```python
from build123d import *

# Parameters (mm, degrees)
SKETCH2_R           = 1.35
BOSS_EXTRUDE1_DEPTH = 36
CIRPATTERN1_COUNT   = 6
CUT_EXTRUDE3_DEPTH  = 36
CUT_EXTRUDE9_DEPTH  = 36


with BuildPart() as part:
    # Sketch2 → Boss-Extrude1 (new body)
    # profile 1 of 10: a face of its own
    with BuildSketch(Plane(origin=(0, 0, 0), x_dir=(1, 0, 0), z_dir=(0, 1, 0))):
        Polygon((-79.212456933, 112.8), (-56.712456933, 73.82885683), (-35.58143708, 86.02885683), (-58.08143708, 125), (0, 125), (0, 0), (-108.253175473, 62.5), align=None)
        with Locations((-77.887328063, 104.904809472)):
            Circle(SKETCH2_R, mode=Mode.SUBTRACT)
        with Locations((-69.387328063, 90.182377607)):
            Circle(SKETCH2_R, mode=Mode.SUBTRACT)
        with Locations((-43.40656595, 105.182377607)):
            Circle(SKETCH2_R, mode=Mode.SUBTRACT)
        with Locations((-51.90656595, 119.904809472)):
            Circle(SKETCH2_R, mode=Mode.SUBTRACT)
        with Locations((-34.90656595, 90.459945743)):
            Circle(SKETCH2_R, mode=Mode.SUBTRACT)
        with Locations((-60.887328063, 75.459945743)):
            Circle(SKETCH2_R, mode=Mode.SUBTRACT)
        with Locations((-52.108162939, 73.253985699)):
            Circle(SKETCH2_R, mode=Mode.SUBTRACT)
        with Locations((-37.385731074, 81.753985699)):
            Circle(SKETCH2_R, mode=Mode.SUBTRACT)
    # profile 2 of 10: a face of its own
    with BuildSketch(Plane(origin=(0, 0, 0), x_dir=(1, 0, 0), z_dir=(0, 1, 0))):
        with Locations((-77.887328063, 104.904809472)):
            Circle(SKETCH2_R)
    # profile 3 of 10: a face of its own
    with BuildSketch(Plane(origin=(0, 0, 0), x_dir=(1, 0, 0), z_dir=(0, 1, 0))):
        with Locations((-69.387328063, 90.182377607)):
            Circle(SKETCH2_R)
    # profile 4 of 10: a face of its own
    with BuildSketch(Plane(origin=(0, 0, 0), x_dir=(1, 0, 0), z_dir=(0, 1, 0))):
        with Locations((-43.40656595, 105.182377607)):
            Circle(SKETCH2_R)
    # profile 5 of 10: a face of its own
    with BuildSketch(Plane(origin=(0, 0, 0), x_dir=(1, 0, 0), z_dir=(0, 1, 0))):
        with Locations((-34.90656595, 90.459945743)):
            Circle(SKETCH2_R)
    # profile 6 of 10: a face of its own
    with BuildSketch(Plane(origin=(0, 0, 0), x_dir=(1, 0, 0), z_dir=(0, 1, 0))):
        with Locations((-37.385731074, 81.753985699)):
            Circle(SKETCH2_R)
    # profile 7 of 10: a face of its own
    with BuildSketch(Plane(origin=(0, 0, 0), x_dir=(1, 0, 0), z_dir=(0, 1, 0))):
        with Locations((-52.108162939, 73.253985699)):
            Circle(SKETCH2_R)
    # profile 8 of 10: a face of its own
    with BuildSketch(Plane(origin=(0, 0, 0), x_dir=(1, 0, 0), z_dir=(0, 1, 0))):
        with Locations((-60.887328063, 75.459945743)):
            Circle(SKETCH2_R)
    # profile 9 of 10: a face of its own
    with BuildSketch(Plane(origin=(0, 0, 0), x_dir=(1, 0, 0), z_dir=(0, 1, 0))):
        with Locations((-51.90656595, 119.904809472)):
            Circle(SKETCH2_R)
    # profile 10 of 10: a face of its own
    with BuildSketch(Plane(origin=(0, 0, 0), x_dir=(1, 0, 0), z_dir=(0, 1, 0))):
        Polygon((-79.212456933, 112.8), (-58.08143708, 125), (-35.58143708, 86.02885683), (-56.712456933, 73.82885683), align=None)
    boss_extrude1 = extrude(amount=BOSS_EXTRUDE1_DEPTH)

    # CirPattern1: Boss-Extrude1 ×6 about axis
    cirpattern1_axis = Axis((0, 0, 0), (0, 1, 0))
    for i in range(1, CIRPATTERN1_COUNT):
        add(boss_extrude1.rotate(cirpattern1_axis, i * 360 / CIRPATTERN1_COUNT))

    # Sketch4 → Cut-Extrude3 (cut)
    with BuildSketch(Plane(origin=(0, 36, 0), x_dir=(1, 0, 0), z_dir=(0, 1, 0))):
        with BuildLine():
            Line((79.212456933, -112.8), (137.293894013, -12.2))
            ThreePointArc((137.293894013, -12.2), (125.5592118, -23.716902798), (109.56410095, -27.524558982))
            ThreePointArc((109.56410095, -27.524558982), (77.942286341, -45), (78.619017782, -81.123015275))
            ThreePointArc((78.619017782, -81.123015275), (83.319046223, -96.879015699), (79.212456933, -112.8))
        make_face()
        with BuildLine():
            Line((137.293894013, 12.2), (79.212456933, 112.8))
            ThreePointArc((79.212456933, 112.8), (83.319046223, 96.879015699), (78.619017782, 81.123015275))
            ThreePointArc((78.619017782, 81.123015275), (77.942286341, 45), (109.56410095, 27.524558982))
            ThreePointArc((109.56410095, 27.524558982), (125.5592118, 23.716902798), (137.293894013, 12.2))
        make_face()
        with BuildLine():
            Line((58.08143708, 125), (-58.08143708, 125))
            ThreePointArc((-58.08143708, 125), (-42.240165578, 120.595918497), (-30.945083169, 108.647574257))
            ThreePointArc((-30.945083169, 108.647574257), (0, 90), (30.945083169, 108.647574257))
            ThreePointArc((30.945083169, 108.647574257), (42.240165578, 120.595918497), (58.08143708, 125))
        make_face()
        with BuildLine():
            Line((-79.212456933, 112.8), (-137.293894013, 12.2))
            ThreePointArc((-137.293894013, 12.2), (-125.5592118, 23.716902798), (-109.56410095, 27.524558982))
            ThreePointArc((-109.56410095, 27.524558982), (-77.942286341, 45), (-78.619017782, 81.123015275))
            ThreePointArc((-78.619017782, 81.123015275), (-83.319046223, 96.879015699), (-79.212456933, 112.8))
        make_face()
        with BuildLine():
            Line((-137.293894013, -12.2), (-79.212456933, -112.8))
            ThreePointArc((-79.212456933, -112.8), (-83.319046223, -96.879015699), (-78.619017782, -81.123015275))
            ThreePointArc((-78.619017782, -81.123015275), (-77.942286341, -45), (-109.56410095, -27.524558982))
            ThreePointArc((-109.56410095, -27.524558982), (-125.5592118, -23.716902798), (-137.293894013, -12.2))
        make_face()
        with BuildLine():
            Line((-58.08143708, -125), (58.08143708, -125))
            ThreePointArc((58.08143708, -125), (42.240165578, -120.595918497), (30.945083169, -108.647574257))
            ThreePointArc((30.945083169, -108.647574257), (0, -90), (-30.945083169, -108.647574257))
            ThreePointArc((-30.945083169, -108.647574257), (-42.240165578, -120.595918497), (-58.08143708, -125))
        make_face()
    extrude(amount=-CUT_EXTRUDE3_DEPTH, mode=Mode.SUBTRACT)

    # Sketch9 → Cut-Extrude9 (cut)
    with BuildSketch(Plane(origin=(0, 36, 0), x_dir=(1, 0, 0), z_dir=(0, 1, 0))):
        with BuildLine():
            ThreePointArc((-30.945083169, 108.647574257), (-41.549939601, 120.167433406), (-56.457326868, 124.956999109))
            ThreePointArc((-56.457326868, 124.956999109), (-49.371438692, 122.503896044), (-44.358314608, 116.927507176))
            ThreePointArc((-44.358314608, 116.927507176), (-25.945860566, 97.258774942), (-5e-08, 90))
            ThreePointArc((-5e-08, 90), (-18.064676866, 95.022217398), (-30.945083169, 108.647574257))
        make_face()
        with BuildLine():
            ThreePointArc((-79.083034312, 96.879180908), (-81.405766691, 104.008868151), (-79.987272175, 111.371978852))
            ThreePointArc((-79.987272175, 111.371978852), (-83.293080236, 96.067019923), (-78.619017782, 81.123015275))
            ThreePointArc((-78.619017782, 81.123015275), (-73.259315749, 63.155577296), (-77.942286796, 44.999999212))
            ThreePointArc((-77.942286796, 44.999999212), (-71.255639547, 71.099161364), (-79.083034312, 96.879180908))
        make_face()
        with BuildLine():
            ThreePointArc((44.358314608, 116.927507176), (49.371438692, 122.503896044), (56.457326868, 124.956999109))
            ThreePointArc((56.457326868, 124.956999109), (41.549939601, 120.167433406), (30.945083169, 108.647574257))
            ThreePointArc((30.945083169, 108.647574257), (18.064676823, 95.022217372), (-5e-08, 90))
            ThreePointArc((-5e-08, 90), (25.945860523, 97.258774916), (44.358314608, 116.927507176))
        make_face()
        with BuildLine():
            ThreePointArc((-109.56410095, 27.524558982), (-124.843019837, 24.100413483), (-136.444599043, 13.585020257))
            ThreePointArc((-136.444599043, 13.585020257), (-130.777205383, 18.495027893), (-123.44134892, 20.048326268))
            ThreePointArc((-123.44134892, 20.048326268), (-97.201500501, 26.159612891), (-77.942286796, 44.999999212))
            ThreePointArc((-77.942286796, 44.999999212), (-91.323993, 31.866639414), (-109.56410095, 27.524558982))
        make_face()
        with BuildLine():
            ThreePointArc((78.619017782, 81.123015275), (83.293080236, 96.067019923), (79.987272175, 111.371978852))
            ThreePointArc((79.987272175, 111.371978852), (81.405766691, 104.008868151), (79.083034312, 96.879180908))
            ThreePointArc((79.083034312, 96.879180908), (71.255639156, 71.099143577), (77.942304587, 44.999968396))
            ThreePointArc((77.942304587, 44.999968396), (73.259315415, 63.155559508), (78.619017782, 81.123015275))
        make_face()
        with BuildLine():
            ThreePointArc((-123.44134892, -20.048326268), (-130.777205383, -18.495027893), (-136.444599043, -13.585020258))
            ThreePointArc((-136.444599043, -13.585020258), (-124.843019837, -24.100413483), (-109.56410095, -27.524558982))
            ThreePointArc((-109.56410095, -27.524558982), (-91.323992191, -31.866639861), (-77.942285871, -45.000000813))
            ThreePointArc((-77.942285871, -45.000000813), (-97.20149969, -26.159613335), (-123.44134892, -20.048326268))
        make_face()
        with BuildLine():
            ThreePointArc((123.44134892, 20.048326268), (130.777205383, 18.495027893), (136.444599043, 13.585020258))
            ThreePointArc((136.444599043, 13.585020258), (124.843019837, 24.100413483), (109.56410095, 27.524558982))
            ThreePointArc((109.56410095, 27.524558982), (91.324008572, 31.866630809), (77.942304587, 44.999968396))
            ThreePointArc((77.942304587, 44.999968396), (97.2015161, 26.159604336), (123.44134892, 20.048326268))
        make_face()
        with BuildLine():
            ThreePointArc((-78.619017782, -81.123015275), (-83.293080236, -96.067019923), (-79.987272175, -111.371978852))
            ThreePointArc((-79.987272175, -111.371978852), (-81.405766691, -104.008868151), (-79.083034312, -96.879180908))
            ThreePointArc((-79.083034312, -96.879180908), (-71.255639567, -71.099162289), (-77.942285871, -45.000000813))
            ThreePointArc((-77.942285871, -45.000000813), (-73.259315766, -63.15557822), (-78.619017782, -81.123015275))
        make_face()
        with BuildLine():
            ThreePointArc((109.56410095, -27.524558982), (124.843019837, -24.100413483), (136.444599043, -13.585020257))
            ThreePointArc((136.444599043, -13.585020257), (130.777205383, -18.495027893), (123.44134892, -20.048326268))
            ThreePointArc((123.44134892, -20.048326268), (97.201499744, -26.159613306), (77.942285932, -45.000000707))
            ThreePointArc((77.942285932, -45.000000707), (91.323992244, -31.866639831), (109.56410095, -27.524558982))
        make_face()
        with BuildLine():
            ThreePointArc((-44.358314608, -116.927507176), (-49.371438692, -122.503896044), (-56.457326868, -124.956999109))
            ThreePointArc((-56.457326868, -124.956999109), (-41.549939601, -120.167433406), (-30.945083169, -108.647574257))
            ThreePointArc((-30.945083169, -108.647574257), (-18.064676844, -95.022217385), (0, -90))
            ThreePointArc((0, -90), (-25.945860545, -97.258774929), (-44.358314608, -116.927507176))
        make_face()
        with BuildLine():
            ThreePointArc((79.083034312, -96.879180908), (81.405766691, -104.008868151), (79.987272175, -111.371978852))
            ThreePointArc((79.987272175, -111.371978852), (83.293080236, -96.067019923), (78.619017782, -81.123015275))
            ThreePointArc((78.619017782, -81.123015275), (73.259315765, -63.155578159), (77.942285932, -45.000000707))
            ThreePointArc((77.942285932, -45.000000707), (71.255639566, -71.099162227), (79.083034312, -96.879180908))
        make_face()
        with BuildLine():
            ThreePointArc((30.945083169, -108.647574257), (41.549939601, -120.167433406), (56.457326867, -124.956999109))
            ThreePointArc((56.457326867, -124.956999109), (49.371438692, -122.503896044), (44.358314608, -116.927507176))
            ThreePointArc((44.358314608, -116.927507176), (25.945860545, -97.258774929), (0, -90))
            ThreePointArc((0, -90), (18.064676844, -95.022217385), (30.945083169, -108.647574257))
        make_face()
    extrude(amount=-CUT_EXTRUDE9_DEPTH, mode=Mode.SUBTRACT)


solid = part.part
```
Geometry: final body of the model. Coordinates: model frame, mm. A direction names the side the tool comes from. Coordinates: 2 decimals unless noted, no trailing zeros. Loops run counter-clockwise (first coordinate to the right, second up) from the corner with the lowest first, then second, coordinate; pieces in that order, holes last. Notation, with made-up numbers: (79.25, 31) -> (125.25, 31) arc R29 cw to (125.25, 62) -> close; hole circle Ø8 at (-32, 28). An arc over 180 degrees is marked (long way). Use a Markdown table: item, result. Add a question column.
(1) Line query: line 1 along Z through (x, y) = (-78, 10.5); line 2 along X through (y, z) = (21, -67.5); line 3 along Z through (x, y) = (-121, 7.5). Output: solid intervals per line, ascending.
(2) Access query for faces 5 (the cylindrical face through (-81.41, 18.25, 104.11)), 6 (the cylindrical face through (-49.283, 18.252, 122.445)), 7 (the cylindrical face through (-49.46, 18.25, -122.56)). Directions: +Z, -Z, +X, -X, +Y, -Y. A direction counts if a zero-diameter tool reaches every point of the face in a straight line with its end or side. Return the directions, or none.
(3) Pin query (flat end, axial travel): pin 1 Ø10 at (y, z) = (10, 59.5) entering from +X; pin 2 Ø10 at (x, y) = (-27, 9) entering from +Z; pin 3 Ø2 at (x, y) = (-13.5, 23.5) entering from -Z. Return the tip coordinate at first contact, or that it passes through.
(4) Section query A-A, the plane z = 106. Return loops of the section in (x, y), plus the area to 3 significant figures.
(5) Section query B-B, the plane x = 99.5. Return loops of the section in (y, z), plus the area to 3 significant figures.
(6) Mould query, pull axis Z, two halves, no side actions, for faces 1 (the cylindrical face through (81.41, 18.25, -104.11)), 2 (the cylindrical face through (-130.682, 18.252, 18.542)), 3 (the flat face through (137.294, 18, 0)), 4 (the flat face through (-68.795, 17.748, -118.815)). Classes: pulls with the +Z half, pulls with the -Z half, needs draft (parallel to the pull), parting line crosses it, or undercut.
(7) Section query C-C, the plane z = -64. Return loops of the section in (x, y), plus the area to 3 significant figures.
Answer:
| question | item | result |
|---|---|---|
| 1 | line 1 | z = -113.5 to -95.1, -44.9 to 44.9, 95.1 to 113.5 |
| 1 | line 2 | x = -71.31 to 71.31 |
| 1 | line 3 | z = -20 to 20 |
| 2 | face 5 | -X, +Y, -Y |
| 2 | face 6 | +Z, +Y, -Y |
| 2 | face 7 | -Z, +Y, -Y |
| 3 | pin 1 | stops at x = 73.71 |
| 3 | pin 2 | stops at z = 101.58 |
| 3 | pin 3 | stops at z = -92.15 |
| 4 | outline | (-81.4, 0) -> (-36.66, 0) -> (-36.66, 36) -> (-81.4, 36) -> close; (36.66, 0) -> (81.4, 0) -> (81.4, 36) -> (36.66, 36) -> close |
| 4 | area | 3,220 mm^2 |
| 5 | outline | (0, -24.98) -> (36, -24.98) -> (36, 24.98) -> (0, 24.98) -> close |
| 5 | area | 1,800 mm^2 |
| 6 | face 1 | undercut |
| 6 | face 2 | pulls with the +Z half |
| 6 | face 3 | needs draft |
| 6 | face 4 | pulls with the -Z half |
| 7 | outline | (-71.6, 0) -> (71.6, 0) -> (71.6, 36) -> (-71.6, 36) -> close |
| 7 | area | 5,160 mm^2 |
